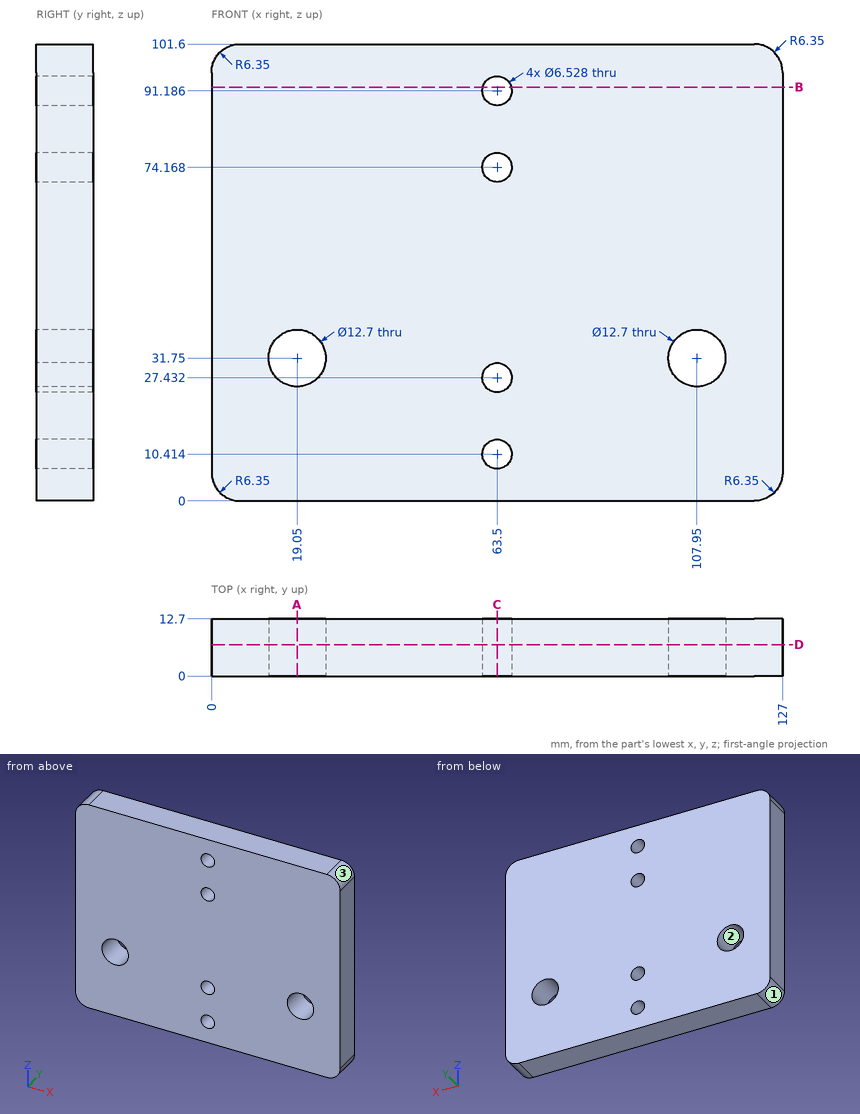
Answer from the drawing. Dimensions are ordinates in mm from the lowest x, y and z of the part. Give positions to 0.01 mm unless a question says otherwise; leave off trailing zeros. Write each loop counter-clockwise with the first axis right and the second up, starting at its lowest first coordinate (ties: lowest second). Pieces come first, ordered by that corner, then holes. Notation, with made-up numbers: (28.5, 89.5) -> (70.5, 89.5) arc R33 cw to (70.5, 117.5) -> close; hole circle Ø5 at (-9, -23.75). An arc over 180 degrees is marked (long way). One line per question, with ' | ' between items. Start each with the question number.
1. Find the intervals of material crossed by probe 1 along X at (y, z) = (9.75, 31.75); probe 2 along X at (y, z) = (2, 91.5); probe 3 along X at (y, z) = (2.25, 29.5) (1 decimal), in increasing order.
2. Section D-D (y = 7) is taken. Determine the outline of the cut face in (x, z).
3. For a pull along X with two mould halves and no side action, classify the marked faces 1, 2 and 3 as pulls with the +X half, pulls with the -X half, needs draft (parallel to the pull), parting line crosses it, or undercut.
4. Section C-C (x = 63.5) is taken. Determine the outline of the cut face in (y, z).
5. Section A-A (x = 19.05) is taken. Determine the outline of the cut face in (y, z), plus the area to 3 significant figures.
6. Section B-B (z = 92) is taken. Determine the outline of the cut face in (x, y), plus the area to 3 significant figures.
Response values:
1) probe 1: 0 to 12.7, 25.4 to 101.6, 114.3 to 127 | probe 2: 0 to 60.25, 66.75 to 127 | probe 3: 0 to 13.1, 25 to 61, 66 to 102, 113.9 to 127
2) outline: (0, 6.35) arc R6.35 ccw to (6.35, 0) -> (120.65, 0) arc R6.35 ccw to (127, 6.35) -> (127, 95.25) arc R6.35 ccw to (120.65, 101.6) -> (6.35, 101.6) arc R6.35 ccw to (0, 95.25) -> close; hole circle Ø12.7 at (19.05, 31.75); hole circle Ø6.53 at (63.5, 10.41); hole circle Ø6.53 at (63.5, 27.43); hole circle Ø6.53 at (63.5, 74.17); hole circle Ø6.53 at (63.5, 91.19); hole circle Ø12.7 at (107.95, 31.75)
3) face 1: pulls with the -X half | face 2: undercut | face 3: pulls with the +X half
4) outline: (0, 0) -> (12.7, 0) -> (12.7, 7.15) -> (0, 7.15) -> close; (0, 13.68) -> (12.7, 13.68) -> (12.7, 24.17) -> (0, 24.17) -> close; (0, 30.7) -> (12.7, 30.7) -> (12.7, 70.9) -> (0, 70.9) -> close; (0, 77.43) -> (12.7, 77.43) -> (12.7, 87.92) -> (0, 87.92) -> close; (0, 94.45) -> (12.7, 94.45) -> (12.7, 101.6) -> (0, 101.6) -> close
5) outline: (0, 0) -> (12.7, 0) -> (12.7, 25.4) -> (0, 25.4) -> close; (0, 38.1) -> (12.7, 38.1) -> (12.7, 101.6) -> (0, 101.6) -> close | area: 1,130 mm2
6) outline: (0, 0) -> (60.34, 0) -> (60.34, 12.7) -> (0, 12.7) -> close; (66.66, 0) -> (127, 0) -> (127, 12.7) -> (66.66, 12.7) -> close | area: 1,530 mm2
